Check sheet for the drawn part. Datum: minimum x, y, z corner. Units: mm. Round coordinates to 2 decimals unless told otherwise and drop trailing zeros. Write each loop counter-clockwise with the first axis right and the second up, starting at its lowest first coordinate (ties: lowest second). Pieces come first, ordered by that corner, then holes.
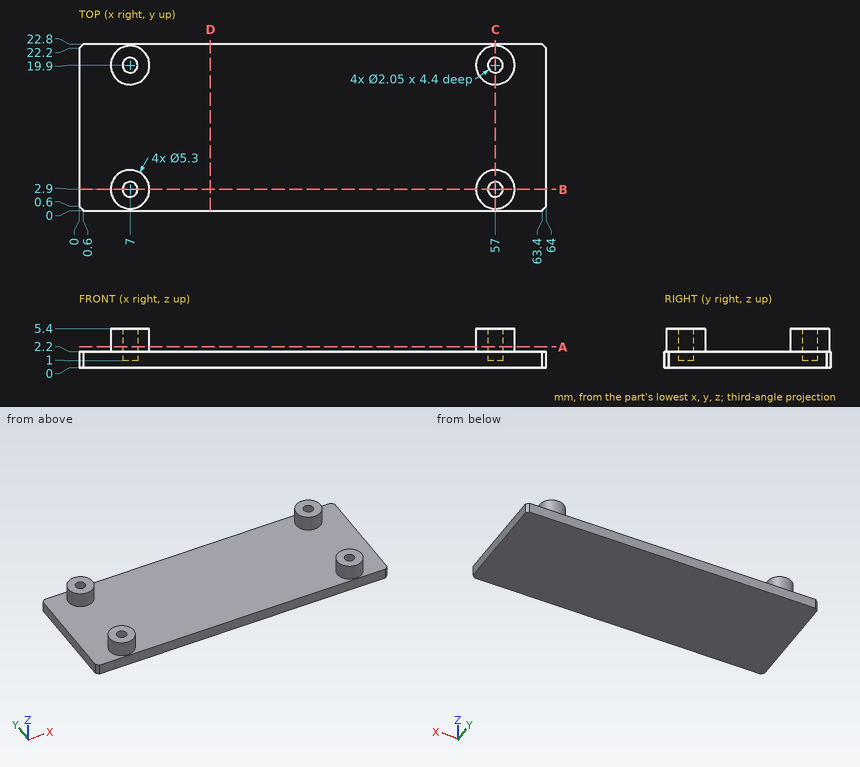
1. Sectioned sample at D-D, the plane x = 18. Enter the section's corners in (y, z).
2. Sectioned sample at B-B, the plane y = 2.9. Enter the section's corners in (x, z) (3 decimals), plus the area to 3 significant figures.
3. Scan lines: line 1 along Y through (x, z) = (57, 2.45) (3 decimals); line 2 along Z through (x, y) = (38, 21); line 3 along X through (y, z) = (3.75, 1.55). Record each from-to range of solid material in increasing order.
4. Go/stop test with flat-tipped pins: pin 1 (1.6 mm diameter, centred on x = 7, y = 2.9, fed in from +Z); pin 2 (7 mm diameter, centred on x = 27, y = 9, fed in from +Z); pin 3 (1 mm diameter, centred on x = 11, z = 4.5, fed in from -Y). Record where each tip stops, or that it passes through.
5. Sectioned sample at C-C, the plane x = 57. Enter the section's corners in (y, z) (3 decimals).
6. Sectioned sample at A-A, the plane z = 2.9. Enter the section's corners in (x, y) (3 decimals).
Computed values:
1. outline: (0, 0) - (22.8, 0) - (22.8, 2.2) - (0, 2.2) - close
2. outline: (0, 0) - (64, 0) - (64, 2.2) - (59.65, 2.2) - (59.65, 5.4) - (58.025, 5.4) - (58.025, 1) - (55.975, 1) - (55.975, 5.4) - (54.35, 5.4) - (54.35, 2.2) - (9.65, 2.2) - (9.65, 5.4) - (8.025, 5.4) - (8.025, 1) - (5.975, 1) - (5.975, 5.4) - (4.35, 5.4) - (4.35, 2.2) - (0, 2.2) - close
2. area: 157 mm2
3. line 1: y = 0.25 to 1.875, 3.925 to 5.55, 17.25 to 18.875, 20.925 to 22.55
3. line 2: z = 0 to 2.2
3. line 3: x = 0 to 6.43, 7.57 to 56.43, 57.57 to 64
4. pin 1: stops at z = 1
4. pin 2: stops at z = 2.2
4. pin 3: passes through
5. outline: (0, 0) - (22.8, 0) - (22.8, 2.2) - (22.55, 2.2) - (22.55, 5.4) - (20.925, 5.4) - (20.925, 1) - (18.875, 1) - (18.875, 5.4) - (17.25, 5.4) - (17.25, 2.2) - (5.55, 2.2) - (5.55, 5.4) - (3.925, 5.4) - (3.925, 1) - (1.875, 1) - (1.875, 5.4) - (0.25, 5.4) - (0.25, 2.2) - (0, 2.2) - close
6. outline: circle Ø5.3 at (7, 2.9); circle Ø5.3 at (7, 19.9); circle Ø5.3 at (57, 2.9); circle Ø5.3 at (57, 19.9); hole circle Ø2.05 at (7, 2.9); hole circle Ø2.05 at (7, 19.9); hole circle Ø2.05 at (57, 2.9); hole circle Ø2.05 at (57, 19.9)
